Answer from the drawing. Dimensions are ordinates in mm from the lowest x, y and z of the part. Round coordinates to 2 decimals unless told otherwise and drop trailing zeros. Order: outer loops, then holes, each group sorted by start corner. A loop starts at its lowest first (then second) coordinate and runs counter-clockwise, first axis right, second up. Notation, with made-up numbers: (81, 87) -> (108, 87) arc R26 ccw to (108, 119) -> close; hole circle Ø11 at (-13.5, 25). An arc over 180 degrees is marked (long way). Use a Markdown table: item, result. Add a question column.
Item 1: A cutting plane is placed at C-C, the plane x = 4. Determine the outline of the cut face in (y, z).
Item 2: A cutting plane is placed at B-B, the plane z = 0.65. Determine the outline of the cut face in (x, y).
Item 3: A cutting plane is placed at D-D, the plane y = 10.75. Determine the outline of the cut face in (x, z).
Item 4: For a pull along Z with two mould halves and no side action, classify the marked faces 1, 2 and 3 as +Z half, -Z half, draft (parallel to the pull), parting line (faces both ways), or undercut.
Item 5: A cutting plane is placed at A-A, the plane y = 6. Determine the outline of the cut face in (x, z).
Item 6: Find the intervals of material crossed by L1, parallel to X at y = 3.25, z = 1.15; L2, parallel to Y at x = 3, z = 3.35; L3, parallel to X at y = 4.25, z = 1.8, in increasing order. Write a range as [from, to].
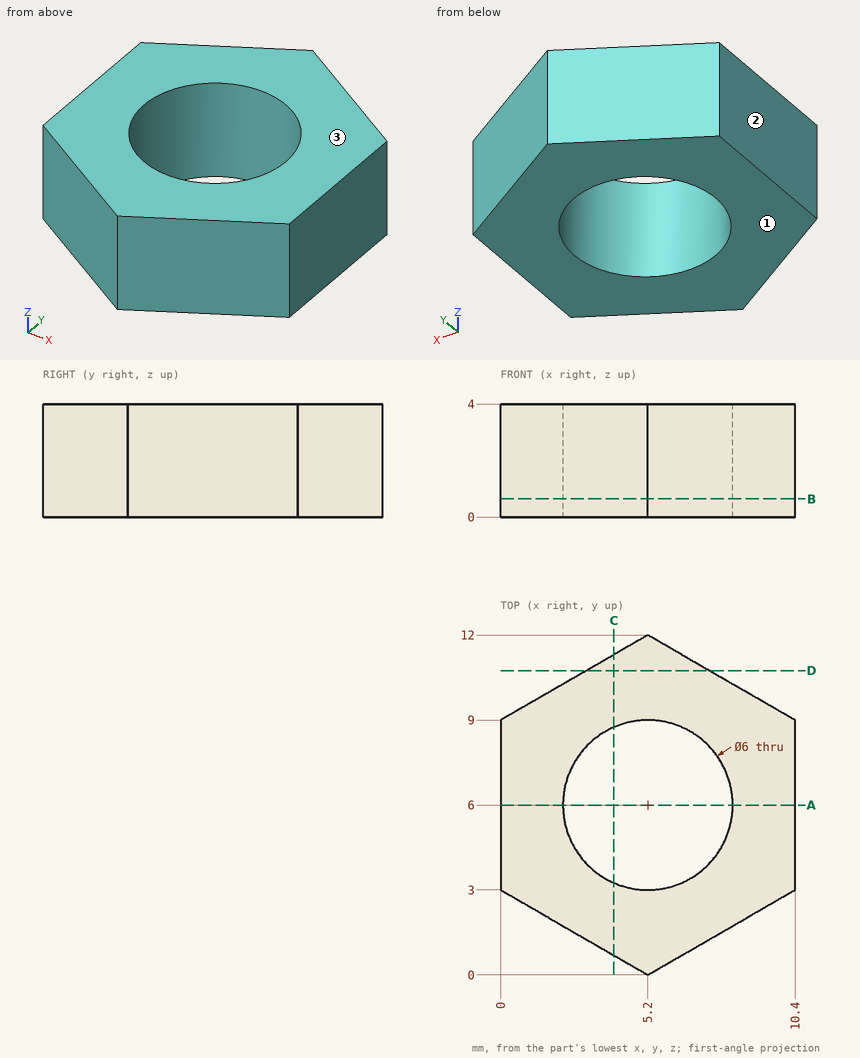
Reported:
| question | item | result |
|---|---|---|
| 1 | outline | (0.69, 0) -> (3.25, 0) -> (3.25, 4) -> (0.69, 4) -> close; (8.75, 0) -> (11.31, 0) -> (11.31, 4) -> (8.75, 4) -> close |
| 2 | outline | (0, 3) -> (5.2, 0) -> (10.4, 3) -> (10.4, 9) -> (5.2, 12) -> (0, 9) -> close; hole circle Ø6 at (5.2, 6) |
| 3 | outline | (3.03, 0) -> (7.37, 0) -> (7.37, 4) -> (3.03, 4) -> close |
| 4 | face 1 | -Z half |
| 4 | face 2 | draft |
| 4 | face 3 | +Z half |
| 5 | outline | (0, 0) -> (2.2, 0) -> (2.2, 4) -> (0, 4) -> close; (8.2, 0) -> (10.4, 0) -> (10.4, 4) -> (8.2, 4) -> close |
| 6 | L1 | [0, 4], [6.4, 10.4] |
| 6 | L2 | [1.27, 3.96], [8.04, 10.73] |
| 6 | L3 | [0, 2.76], [7.64, 10.4] |
